```python
from build123d import *

# Parameters (mm, degrees)
BOSS_EXTRUDE1_DEPTH = 15
SKETCH3_W           = 25
SKETCH3_H           = 3
BOSS_EXTRUDE2_DEPTH = 5


with BuildPart() as part:
    # Sketch2 → Boss-Extrude1 (new body)
    with BuildSketch(Plane.XY):
        Polygon((0, 0), (0, 25.4), (-2.5, 25.4), (-5, 10), (-5, 0), align=None)
    extrude(amount=BOSS_EXTRUDE1_DEPTH)

    # Sketch3 → Boss-Extrude2 (add)
    with BuildSketch(Plane.XZ):
        with Locations((7.5, 1.5)):
            Rectangle(SKETCH3_W, SKETCH3_H)
    extrude(amount=BOSS_EXTRUDE2_DEPTH)


solid = part.part
```
The listing builds one solid part. Answer for the finished solid, in the listing's coordinates (mm). A direction names the side the tool comes from. Coordinates: 2 decimals unless noted, no trailing zeros. Write each loop counter-clockwise with the first axis right and the second up, starting at its lowest first coordinate (ties: lowest second). Pieces come first, ordered by that corner, then holes.
Q1. Section C-C, the plane y = 2.5 is taken. Write down the section's boundary in (x, z).
Returned:
outline: (-5, 0) - (0, 0) - (0, 15) - (-5, 15) - close
Q2. Section A-A, the plane z = 6.5 is taken. Write down the section's boundary in (x, y), then the cut area to 3 significant figures.
Returned:
outline: (-5, 0) - (0, 0) - (0, 25.4) - (-2.5, 25.4) - (-5, 10) - close
area: 108 mm2
Q3. Given P1, Ø4, axis at x = 3, y = -2.5, coming from the +Z side; P2, Ø3, axis at x = 0.5, z = 9.5, coming from the -Y side; P3, Ø12, axis at x = 2, y = 16, coming from the +Z side; P4, Ø2, axis at y = -0.5, z = 7.5, coming from the +X side, each flat-ended and moving along its own axis, determine where each tip first touches the part or whether it passes through.
Returned:
P1: stops at z = 3
P2: stops at y = 0
P3: stops at z = 15
P4: stops at x = 0
Q4. Find the intervals of material crossed by line 1 along Y through (x, z) = (7, 1.25); line 2 along Z through (x, y) = (2.5, -1), in increasing order.
Returned:
line 1: y = -5 to 0
line 2: z = 0 to 3
Q5. Which of the six approach directions +Z, -Z, +X, -X, +Y, -Y give full straight-line access (tool end or side, diameter ignored) to faces 1 (the flat face through (-5, 4, 7)), 2 (the flat face through (7, -2, 3)), 3 (the flat face through (10, 0, 2))?
Returned:
face 1: +Z, -Z, -X, +Y, -Y
face 2: +Z, +X, -X, -Y
face 3: +Z, -Z, +X, +Y
Q6. Section B-B, the plane x = 2.5 is taken. Write down the section's boundary in (y, z), then the cut area to 3 significant figures.
Returned:
outline: (-5, 0) - (0, 0) - (0, 3) - (-5, 3) - close
area: 15.0 mm2
